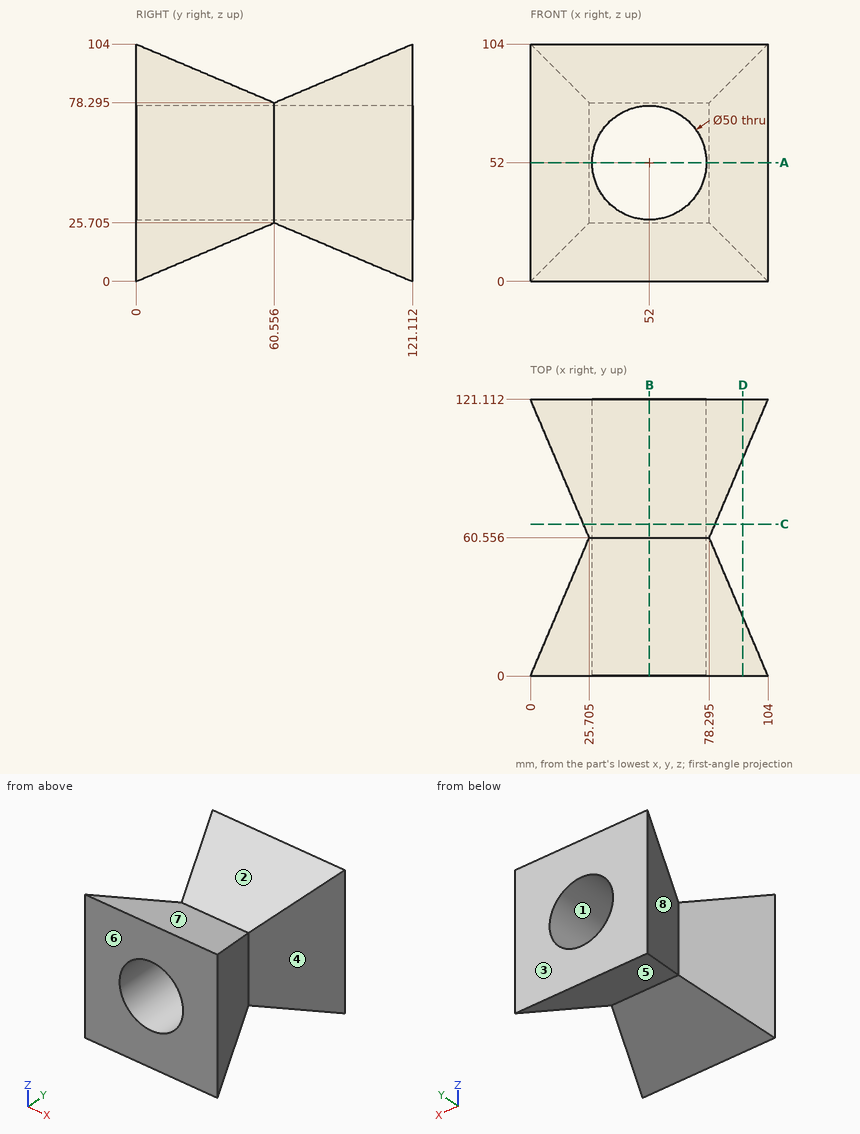
Input: dimensioned drawing with shaded views. Units: mm. Origin: part minimum x, y, z. A direction names the side the tool comes from. Round coordinates to 2 decimals unless told otherwise and drop trailing zeros. Order: outer loops, then holes, each group sorted by start corner. A loop starts at its lowest first (then second) coordinate and runs counter-clockwise, first axis right, second up. Notation, with made-up numbers: (2, -20.75) - (41, -20.75) arc R21 ccw to (41, 15.25) - close; hole circle Ø11 at (37.5, 31). An arc over 180 degrees is marked (long way). Use CSV: the item, a comma, the result in double quotes. Start each with the question number.
Q1. Section query C-C (y = 66.5). Return loops of the section in (x, z), and give its area (3 significant figures).
Q2. Material intervals for line 1 along Z through (x, y) = (42, 19) (1 decimal); line 2 along X through (y, z) = (37.5, 65.5); line 3 along X through (y, z) = (23, 30) (1 decimal), sorted ascending. Write a range as from..to.
Q3. Section query A-A (z = 52). Return loops of the section in (x, y) (1 decimal).
Q4. First-contact query: pin 1 (4 mm diameter, centred on y = 35.5, z = 68, fed in from +X); pin 2 (10 mm diameter, centred on x = 67.5, y = 18.5, fed in from +Z); pin 3 (1.5 mm diameter, centred on y = 57.5, z = 30.5, fed in from -X). Flat tips, straight axial feed; report the tip coordinate or a pass-through.
Q5. Mould query, pull axis Y, two halves, no side actions, for the marked faces 1, 2 and 3. Classes: +Y half, -Y half, draft (parallel to the pull), parting line (faces both ways), or undercut.
Q6. Access query for the marked faces 4, 5, 6, 7 and 8. Directions: +Z, -Z, +X, -X, +Y, -Y. A direction counts if a zero-diameter tool reaches every point of the face in a straight line with its end or side. Return the directions, or none.
Q7. Section query D-D (x = 93). Return loops of the section in (y, z) (1 decimal).
Q8. Section query B-B (x = 52). Return loops of the section in (y, z) (1 decimal).
Result set:
1,outline,"(23.18, 23.18) - (80.82, 23.18) - (80.82, 80.82) - (23.18, 80.82) - close; hole circle Ø50 at (52, 52)"
1,area,"1,360 mm2"
2,line 1,"z = 8.1..29.1, 74.9..95.9"
2,line 2,"x = 15.92..30.96, 73.04..88.08"
2,line 3,"x = 9.8..40.1, 63.9..94.2"
3,outline,"(0, 0) - (27, 0) - (27, 121.1) - (0, 121.1) - (25.7, 60.6) - close; (77, 0) - (104, 0) - (78.3, 60.6) - (104, 121.1) - (77, 121.1) - close"
4,pin 1,"stops at x = 89.78"
4,pin 2,"stops at z = 98.27"
4,pin 3,"stops at x = 24.09"
5,face 1,"draft"
5,face 2,"undercut"
5,face 3,"+Y half"
6,face 4,"+Z, -Z, +X"
6,face 5,"-Z, +X, -X"
6,face 6,"+Z, -Z, +X, -X, -Y"
6,face 7,"+Z, +X, -X"
6,face 8,"+Z, -Z, -X"
7,outline,"(0, 0) - (25.9, 11) - (25.9, 93) - (0, 104) - close; (95.2, 11) - (121.1, 0) - (121.1, 104) - (95.2, 93) - close"
8,outline,"(0, 0) - (60.6, 25.7) - (121.1, 0) - (121.1, 27) - (0, 27) - close; (0, 77) - (121.1, 77) - (121.1, 104) - (60.6, 78.3) - (0, 104) - close"
